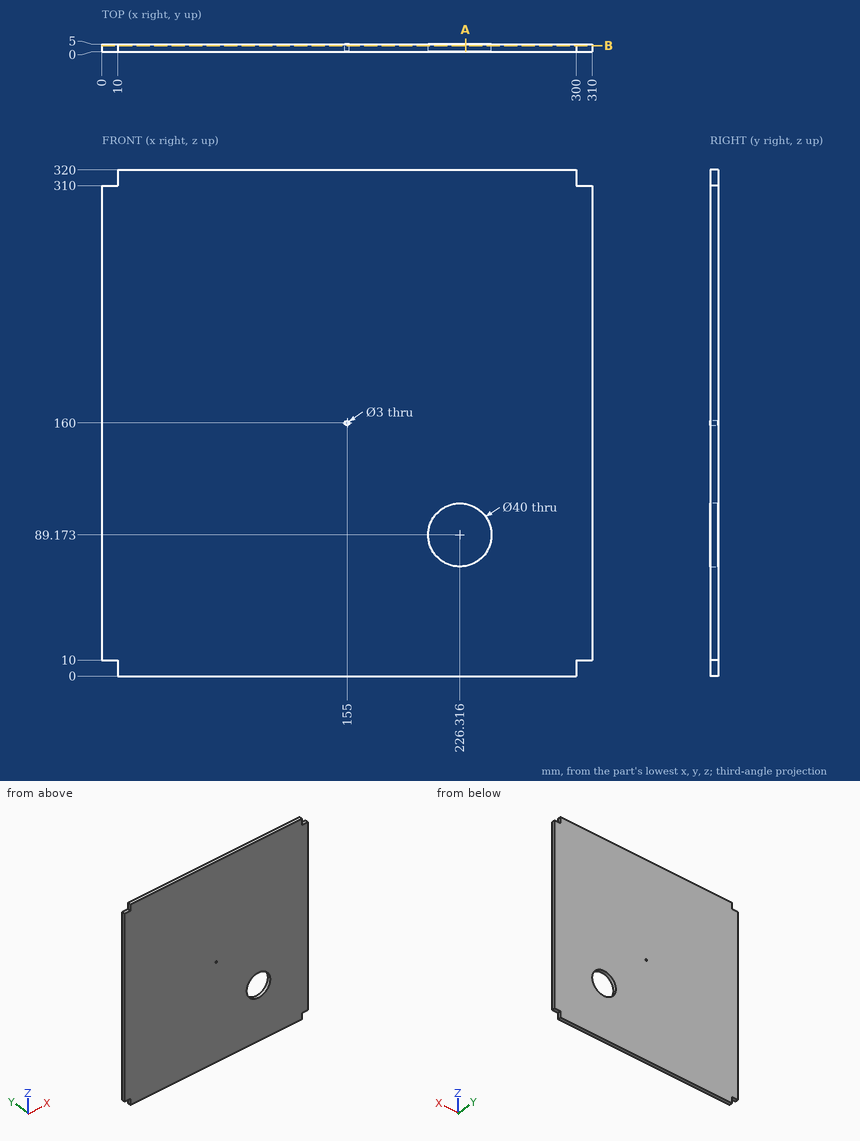
Geometry: see drawing. Coordinates: mm, zero at the bounding-box minimum. Give positions to 0.01 mm unless a question says otherwise; leave off trailing zeros. Order: outer loops, then holes, each group sorted by start corner. A loop starts at its lowest first (then second) coordinate and runs counter-clockwise, first axis right, second up. Notation, with made-up numbers: (64, -28) - (70, -28) arc R6 ccw to (70, -23) - close; hole circle Ø10 at (-35, 50.5). An arc over 180 degrees is marked (long way). Use a Markdown table: item, result.
(1) Section query B-B (y = 3.9). Output: boundary loops of the cut face in (x, z) (1 decimal).
Computed values:
| item | result |
|---|---|
| outline | (0, 10) - (10, 10) - (10, 0) - (300, 0) - (300, 10) - (310, 10) - (310, 310) - (300, 310) - (300, 320) - (10, 320) - (10, 310) - (0, 310) - close; hole circle Ø3 at (155, 160); hole circle Ø40 at (226.3, 89.2) |
(2) Pin query (flat end, axial travel): pin 1 (2.5 mm diameter, centred on y = 1.5, z = 6, fed in from +X); pin 2 (1.5 mm diameter, centred on x = 7, y = 2, fed in from +Z). Return the tip coordinate at first contact, or that it passes through.
Computed values:
| item | result |
|---|---|
| pin 1 | stops at x = 300 |
| pin 2 | stops at z = 310 |
(3) Line query: line 1 (Z direction, x = 155, y = 1); line 2 (Z direction, x = 226, y = 1.8); line 3 (X direction, y = 3.25, z = 160). Output: solid intervals per line, ascending. Write a range as from..to.
Computed values:
| item | result |
|---|---|
| line 1 | z = 0..158.5, 161.5..320 |
| line 2 | z = 0..69.18, 109.17..320 |
| line 3 | x = 0..153.5, 156.5..310 |
(4) Section query A-A (x = 230). Output: boundary loops of the cut face in (y, z) (1 decimal).
Computed values:
| item | result |
|---|---|
| outline | (0, 0) - (5, 0) - (5, 69.5) - (0, 69.5) - close; (0, 108.8) - (5, 108.8) - (5, 320) - (0, 320) - close |
